Verification items for this drawing (mm, ordinates from the low corner). Round coordinates to 2 decimals unless told otherwise and drop trailing zeros. Order: outer loops, then holes, each group sorted by start corner. A loop starts at its lowest first (then second) coordinate and runs counter-clockwise, first axis right, second up. Notation, with made-up numbers: (42.25, 6) - (59.25, 6) arc R26 cw to (59.25, 34) - close; hole circle Ø6 at (37, 72). An arc over 180 degrees is marked (long way). Return JSON: item names as keys, results as strings. Group by question number.
Q1. Sectioned sample at B-B, the plane x = 144.5. Record the cut outline in (y, z).
Q2. Gauge pin test, flat end, axial feed: pin 1 Ø6 at (x, z) = (314, 61) entering from -Y. Record the tip position at first contact, or that the pin passes through.
Q3. Draft check along Z on the marked faces 1, 2, 3 and 4. Enter one of: pulls with the +Z half, pulls with the -Z half, needs draft (parallel to the pull), parting line crosses it, or undercut.
Q4. Material ranges on line 1 along X through (y, z) = (20.25, 102.5); line 2 along Z through (x, y) = (245, 6.75); line 3 along Z through (x, y) = (82, 12.5) (1 decimal), recorded low to high.
Q5. Sectioned sample at C-C, the plane z = 64. Record the cut outline in (x, y).
Q6. Sectioned sample at A-A, the plane y = 12.75. Record the cut outline in (x, z) (1 decimal), then the cut area to 3 significant figures.
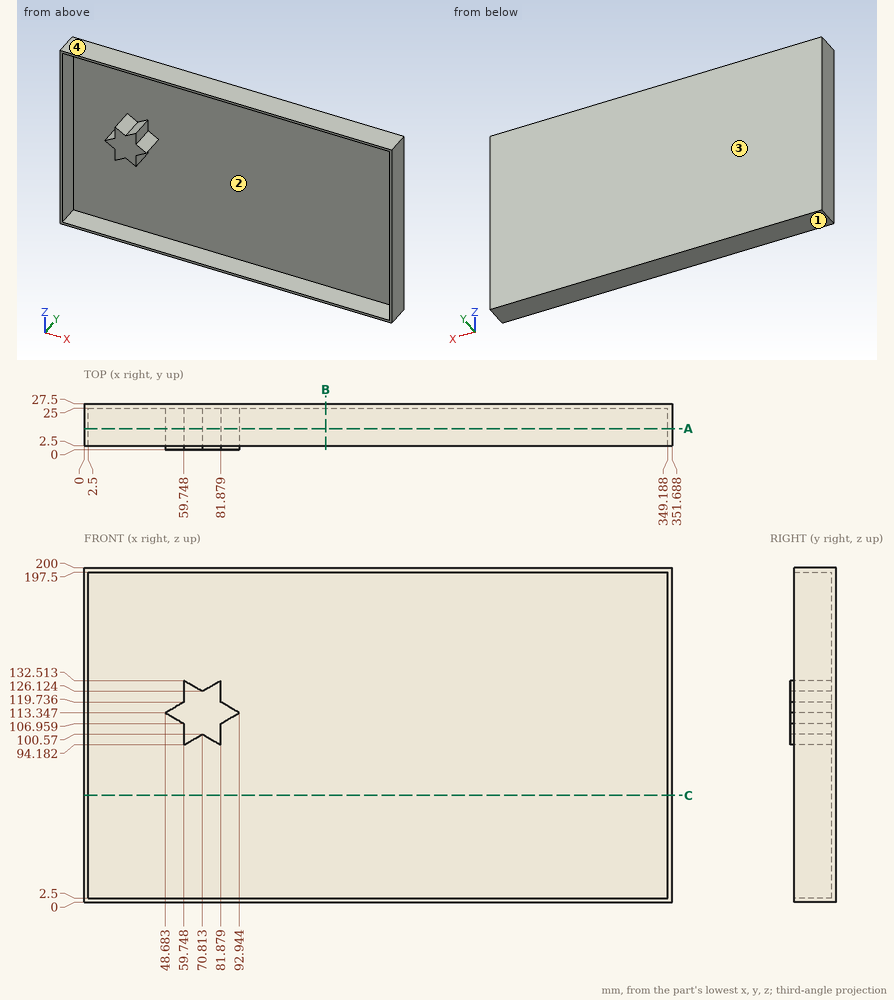
Reply:
{
 "1": {"outline": "(2.5, 0) - (27.5, 0) - (27.5, 200) - (2.5, 200) - (2.5, 197.5) - (25, 197.5) - (25, 2.5) - (2.5, 2.5) - close"},
 "2": {"pin 1": "y = 25"},
 "3": {"face 1": "pulls with the -Z half", "face 2": "undercut", "face 3": "needs draft", "face 4": "pulls with the +Z half"},
 "4": {"line 1": "0 to 2.5, 59.75 to 81.88, 349.19 to 351.69", "line 2": "0 to 2.5, 197.5 to 200", "line 3": "0 to 2.5, 107 to 119.7, 197.5 to 200"},
 "5": {"outline": "(0, 2.5) - (2.5, 2.5) - (2.5, 25) - (349.19, 25) - (349.19, 2.5) - (351.69, 2.5) - (351.69, 27.5) - (0, 27.5) - close"},
 "6": {"outline": "(0, 0) - (351.7, 0) - (351.7, 200) - (0, 200) - close; (48.7, 113.3) - (59.7, 107) - (59.7, 94.2) - (70.8, 100.6) - (81.9, 94.2) - (81.9, 107) - (92.9, 113.3) - (81.9, 119.7) - (81.9, 132.5) - (70.8, 126.1) - (59.7, 132.5) - (59.7, 119.7) - close; hole (2.5, 2.5) - (349.2, 2.5) - (349.2, 197.5) - (2.5, 197.5) - close", "area": "3,580 mm^2"}
}
